Geometry check sheet. Reference: the model listing, model coordinates, mm. A direction names the side the tool comes from. Coordinates: 2 decimals unless noted, no trailing zeros. Write each loop counter-clockwise with the first axis right and the second up, starting at its lowest first coordinate (ties: lowest second). Pieces come first, ordered by that corner, then holes. Notation, with made-up numbers: (63, 3.25) -> (79, 3.25) arc R32 ccw to (79, 36.25) -> close; hole circle Ø9 at (86.25, 40.5). An arc over 180 degrees is marked (long way). Use a Markdown table: item, result.
```python
from build123d import *


with BuildPart() as f2:
    # F1 (on Right) → F2 (revolve)
    with BuildSketch(Plane.YZ):
        Polygon((-30, 0), (30, 0), (30, 100), (30, 350.3538290725), (66, 360), (66, 405), (46, 405), (37.9615242271, 375), (0, 375), (-37.9615242271, 375), (-46, 405), (-66, 405), (-66, 360), (-30, 350.3538290725), (-30, 100), align=None)
        Polygon((30, 100), (30, 0), (106, 0), (106, 79.6358613752), align=None)
        Polygon((-106, 0), (-30, 0), (-30, 100), (-106, 79.6358613752), align=None)
    revolve(axis=Axis((0, 0, 0), (0, -1, 0)))


solid = f2.part
```
Item 1: Depth check by flat-ended pin: P1, Ø6, axis at x = 259, z = -266.5, coming from the +Y side; P2, Ø3, axis at x = 226, z = -31.5, coming from the +Y side; P3, Ø10, axis at x = 90, y = 33, coming from the -Z side; P4, Ø12, axis at x = -182, y = 76, coming from the -Z side. Enter the tip coordinate at first touch or a pass-through.
Answer block:
| item | result |
|---|---|
| P1 | stops at y = 66 |
| P2 | stops at y = 30 |
| P3 | stops at z = -365.24 |
| P4 | passes through |
Item 2: Section check A-A on x = 0. Record the boundary of the cut face in (y, z).
Answer block:
| item | result |
|---|---|
| outline | (-106, -79.64) -> (-30, -100) -> (-30, -350.35) -> (-66, -360) -> (-66, -405) -> (-46, -405) -> (-37.96, -375) -> (37.96, -375) -> (46, -405) -> (66, -405) -> (66, -360) -> (30, -350.35) -> (30, -100) -> (106, -79.64) -> (106, 79.64) -> (30, 100) -> (30, 350.35) -> (66, 360) -> (66, 405) -> (46, 405) -> (37.96, 375) -> (-37.96, 375) -> (-46, 405) -> (-66, 405) -> (-66, 360) -> (-30, 350.35) -> (-30, 100) -> (-106, 79.64) -> close |
Item 3: Mould release check, pull along X, two halves, no side actions. Record for faces 4 (the cylindrical face through (155.117, 55.86, 374.117)), 5 (the flat face through (238, 66, 272)), 6 (the conical face through (80.9, -93.9, -18)): +X half, -X half, draft (parallel to the pull), parting line (faces both ways), or undercut.
Answer block:
| item | result |
|---|---|
| face 4 | parting line |
| face 5 | draft |
| face 6 | undercut |
Item 4: Tool access check on faces 1 (the conical face through (229.07, 38.35, -298.74)), 2 (the flat face through (73, 30, -73)), 3 (the flat face through (73, -30, 73)). Record the directions out of +Z, -Z, +X, -X, +Y, -Y that give a thin tool (end or side, any length) a straight path to the whole face; none if there is none.
Answer block:
| item | result |
|---|---|
| face 1 | none |
| face 2 | +Y |
| face 3 | -Y |
Item 5: Thickness scan on L1, parallel to Z at x = -77.5, y = -53; L2, parallel to Z at x = 41, y = 47; L3, parallel to X at y = 36.5, z = 33. Record the ranges inside material, lowest first. Write a range as [from, to].
Answer block:
| item | result |
|---|---|
| L1 | z = [-397.52, -347.99], [-52.91, 52.91], [347.99, 397.52] |
| L2 | z = [-402.92, -352.53], [-86.19, 86.19], [352.53, 402.92] |
| L3 | x = [-373.55, -350.55], [-92.55, 92.55], [350.55, 373.55] |
Item 6: Section check B-B on z = 0. Record the boundary of the cut face in (x, y), then the cut area to 3 significant figures.
Answer block:
| item | result |
|---|---|
| outline | (-405, -66) -> (-360, -66) -> (-350.35, -30) -> (-100, -30) -> (-79.64, -106) -> (79.64, -106) -> (100, -30) -> (350.35, -30) -> (360, -66) -> (405, -66) -> (405, -46) -> (375, -37.96) -> (375, 37.96) -> (405, 46) -> (405, 66) -> (360, 66) -> (350.35, 30) -> (100, 30) -> (79.64, 106) -> (-79.64, 106) -> (-100, 30) -> (-350.35, 30) -> (-360, 66) -> (-405, 66) -> (-405, 46) -> (-375, 37.96) -> (-375, -37.96) -> (-405, -46) -> close |
| area | 78,000 mm^2 |
